Build history of the part. All positions in model axes, mm. Face numbers are marked on the shaded views. A direction names the side the tool comes from. Round coordinates to 2 decimals unless told otherwise and drop trailing zeros. Loops run counter-clockwise (first coordinate to the right, second up) from the corner with the lowest first, then second, coordinate; pieces in that order, holes last.
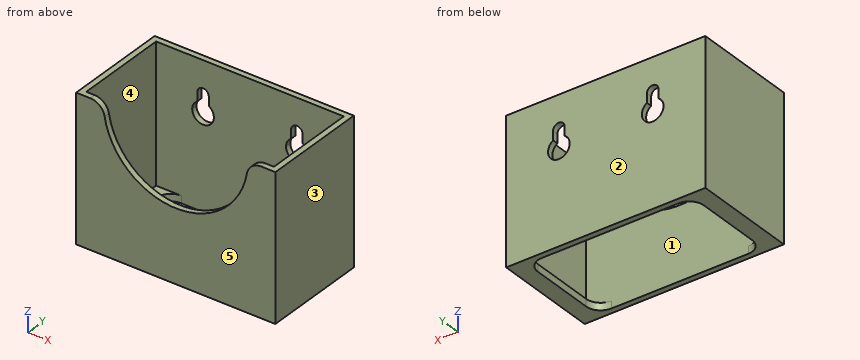
from build123d import *

# Parameters (mm, degrees)
F0_W     = 70.104
F0_H     = 37.084
F0_W_2   = 66.04
F0_H_2   = 33.02
F1_DEPTH = 50.8
F2_DEPTH = 2.54
F3_W     = 58.42
F3_H     = 33.02
F4_DEPTH = 25.4
F6_DEPTH = 25.4
F8_DEPTH = 25.4
F9_R     = 5.08


with BuildPart() as f1:
    # F0 (on Top) → F1 (new body)
    with BuildSketch(Plane.XY):
        with Locations((33.02, 16.51)):
            Rectangle(F0_W, F0_H)
        with Locations((33.02, 16.51)):
            Rectangle(F0_W_2, F0_H_2, mode=Mode.SUBTRACT)
    extrude(amount=F1_DEPTH)

    # F0 (on Top) → F2 (join)
    with BuildSketch(Plane.XY):
        with Locations((33.02, 16.51)):
            Rectangle(F0_W_2, F0_H_2)
    extrude(amount=F2_DEPTH)

    # F3 (on face) → F4 (cut)
    with BuildSketch(Plane.XY.offset(2.54)):
        with Locations((33.02, 16.51)):
            Rectangle(F3_W, F3_H)
    extrude(amount=-F4_DEPTH, mode=Mode.SUBTRACT)

    # F5 (on face) → F6 (cut)
    with BuildSketch(Plane.XZ.offset(2.032)):
        with BuildLine():
            Line((58.42, 50.8), (7.62, 50.8))
            ThreePointArc((7.62, 50.8), (33.02, 25.4), (58.42, 50.8))
        make_face()
    extrude(amount=-F6_DEPTH, mode=Mode.SUBTRACT)

    # F7 (on face) → F8 (cut)
    with BuildSketch(Plane(origin=(0, 35.052, 0), x_dir=(-1, 0, 0), z_dir=(0, 1, 0))):
        with BuildLine():
            ThreePointArc((-51.562, 36.2428986953), (-51.3704048468, 29.6839829137), (-45.72, 33.02))
            ThreePointArc((-45.72, 33.02), (-46.1939829137, 34.8604048468), (-47.498, 36.2428986953))
            ThreePointArc((-47.498, 36.2428986953), (-49.53, 36.83), (-51.562, 36.2428986953))
        make_face()
        with BuildLine():
            ThreePointArc((-51.562, 36.2428986953), (-49.53, 36.83), (-47.498, 36.2428986953))
            Line((-47.498, 36.2428986953), (-47.498, 39.37))
            ThreePointArc((-47.498, 39.37), (-49.53, 41.402), (-51.562, 39.37))
            Line((-51.562, 39.37), (-51.562, 36.2428986953))
        make_face()
        with BuildLine():
            ThreePointArc((-18.542, 36.2428986953), (-16.51, 36.83), (-14.478, 36.2428986953))
            Line((-14.478, 36.2428986953), (-14.478, 39.37))
            ThreePointArc((-14.478, 39.37), (-16.51, 41.402), (-18.542, 39.37))
            Line((-18.542, 39.37), (-18.542, 36.2428986953))
        make_face()
        with BuildLine():
            ThreePointArc((-18.542, 36.2428986953), (-18.3504048468, 29.6839829137), (-12.7, 33.02))
            ThreePointArc((-12.7, 33.02), (-13.1739829137, 34.8604048468), (-14.478, 36.2428986953))
            ThreePointArc((-14.478, 36.2428986953), (-16.51, 36.83), (-18.542, 36.2428986953))
        make_face()
    extrude(amount=-F8_DEPTH, mode=Mode.SUBTRACT)

    # F9
    f9_edges = [f1.edges().sort_by_distance(p)[0] for p in [
        (58.42, -1.016, 50.8),
        (7.62, -1.016, 50.8),
        (62.23, 0, 1.27),
        (62.23, 33.02, 1.27),
        (3.81, 33.02, 1.27),
        (3.81, 0, 1.27),
    ]]
    fillet(f9_edges, radius=F9_R)


solid = f1.part
(1) Slice it at B-B on x = 17. List the corners of the cut face in (y, z), plus the area to 3 significant figures.
Responses:
outline: (-2.03, 0) - (0, 0) - (0, 31.09) - (-2.03, 31.09) - close; (33.02, 0) - (35.05, 0) - (35.05, 29.24) - (33.02, 29.24) - close; (33.02, 41.34) - (35.05, 41.34) - (35.05, 50.8) - (33.02, 50.8) - close
area: 142 mm2
(2) Which spindle directions (+Z, -Z, +X, -X, +Y, -Y) get a long thin tool onto all of the face, cutting with end or side? Do the marked faces 4 and 5. Say none if no direction does.
Responses:
face 4: +Z
face 5: +Z, -Z, +X, -X, -Y
(3) Slice it at A-A on y = 6. List the corners of the cut face in (x, z).
Responses:
outline: (-2.03, 0) - (3.81, 0) - (3.81, 2.54) - (0, 2.54) - (0, 50.8) - (-2.03, 50.8) - close; (62.23, 0) - (68.07, 0) - (68.07, 50.8) - (66.04, 50.8) - (66.04, 2.54) - (62.23, 2.54) - close
(4) Probe line 1 (X direction, y = 34.4, z = 33.02); line 2 (Y direction, x = 50, z = 3); line 3 (X direction, y = 16.5, z = 24). List the from-to ranges inside material, lowest first.
Responses:
line 1: x = -2.03 to 12.7, 20.32 to 45.72, 53.34 to 68.07
line 2: y = -2.03 to 0, 33.02 to 35.05
line 3: x = -2.03 to 0, 66.04 to 68.07
(5) Slice it at D-D on z = 21.5. List the corners of the cut face in (x, y).
Responses:
outline: (-2.03, -2.03) - (68.07, -2.03) - (68.07, 35.05) - (-2.03, 35.05) - close; hole (0, 0) - (66.04, 0) - (66.04, 33.02) - (0, 33.02) - close
(6) Pin check, flat tip, straight feed: P1, Ø7, axis at x = 6.5, y = 9, coming from the +Z side. Stop position of the tip, or through.
Responses:
P1: stops at z = 2.54
(7) Slice it at C-C on z = 35. List the corners of the cut face in (x, y), plus the area to 3 significant figures.
Responses:
outline: (-2.03, -2.03) - (13.13, -2.03) - (13.13, 0) - (0, 0) - (0, 33.02) - (13.25, 33.02) - (13.25, 35.05) - (-2.03, 35.05) - close; (19.77, 33.02) - (46.27, 33.02) - (46.27, 35.05) - (19.77, 35.05) - close; (52.79, 33.02) - (66.04, 33.02) - (66.04, 0) - (52.91, 0) - (52.91, -2.03) - (68.07, -2.03) - (68.07, 35.05) - (52.79, 35.05) - close
area: 312 mm2
(8) Pull direction X, two halves, no side cores. Call the marked faces 1, 2 and 3: +X half, -X half, draft (parallel to the pull), parting line (faces both ways), or undercut.
Responses:
face 1: undercut
face 2: draft
face 3: +X half
